Read the model definition and answer for the solid it produces. Units are mm, in the model's axes. Face numbers are marked on the shaded views. A direction names the side the tool comes from. Coordinates: 2 decimals unless noted, no trailing zeros. Loops run counter-clockwise (first coordinate to the right, second up) from the corner with the lowest first, then second, coordinate; pieces in that order, holes last. Notation, with made-up numbers: (63.25, 36) -> (71.25, 36) arc R18 ccw to (71.25, 41) -> close; hole circle Ø7 at (56.25, -1). An arc over 180 degrees is marked (long way). Answer as a JSON object with one key per item and string values. Group by question number.
Q1. The part is cut by section D-D on x = 9. Write down the section's boundary in (y, z), and give its area (3 significant figures).
Q2. Straight lines are drawn through the part: line 1 along X through (y, z) = (0.5, 1.25) (3 decimals); line 2 along Z through (x, y) = (7.25, 6.25); line 3 along X through (y, z) = (-2.5, -5.25) (3 decimals). For each, find the intervals that lie inside material, in ascending order. Write a range as [from, to].
Q3. Determine the mould class of the marked faces 1, 2 and 3 for opening direction X: released by +X, released by -X, zero draft, split by the parting line, or undercut.
Q4. For the marked faces 4, 5 and 6, determine the directions among +Z, -Z, +X, -X, +Y, -Y from which every point of the face is accessible in a straight line to the end or side of a thin tool.
Q5. The part is cut by section A-A on z = 1. Write down the section's boundary in (x, y) (3 decimals), and give its area (3 significant figures).
Q6. The part is cut by section C-C on y = 3. Write down the section's boundary in (x, z) (3 decimals), and give its area (3 significant figures).
Q7. Each of these flat-tipped pins is pushed along its axis until it touches: P1, Ø3, axis at x = 9, y = 4.5, coming from the +Z side; P2, Ø1.1, axis at x = -12, z = 1, coming from the +Y side (3 decimals); P3, Ø1.5, axis at x = 12, z = 1.5, coming from the -Y side (3 decimals). Where does it stop, or does it pass through?
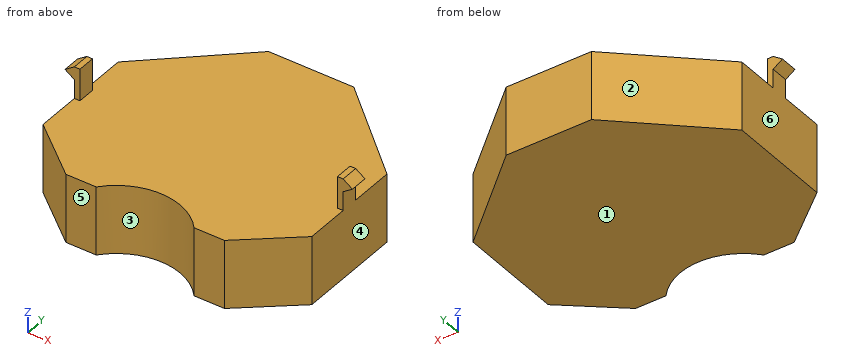
from build123d import *

# Parameters (mm, degrees)
F1_DEPTH      = 6.1
F3_DEPTH      = 0.785
F3_DEPTH_BACK = 0.785
F5_DEPTH      = 8.931
F6_ANGLE      = 180


with BuildPart() as f1:
    # F0 (on Top) → F1 (new body)
    with BuildSketch(Plane.XY):
        Polygon((-7.0355, 8.75), (-11.925, 4.7117), (-11.925, -4.7117), (-3.785, -12.05), (3.785, -12.05), (11.925, -4.7117), (11.925, 4.7117), (7.0355, 8.75), align=None)
    extrude(amount=F1_DEPTH)

    # F2 (on Front) → F3 (join, two sides)
    with BuildSketch(Plane.XZ) as f3_sk:
        Polygon((-11.425, 0), (-11.925, 0), (-11.925, -1.6852878034), (-12.75, -2.2576439017), (-11.925, -2.83), (-11.425, -2.83), align=None)
        Polygon((11.925, -1.6852878034), (11.925, 0), (11.425, 0), (11.425, -2.83), (11.925, -2.83), (12.75, -2.2576439017), align=None)
    extrude(amount=F3_DEPTH)
    extrude(f3_sk.sketch, amount=-F3_DEPTH_BACK)

    # F4 (on face) → F5 (cut, through all)
    with BuildSketch(Plane.XY.offset(6.1)):
        with BuildLine():
            Line((4.342041453, 8.75), (-4.342041453, 8.75))
            ThreePointArc((-4.342041453, 8.75), (0, 6.7139288477), (4.342041453, 8.75))
        make_face()
    extrude(amount=-F5_DEPTH, mode=Mode.SUBTRACT)


with BuildPart() as f1_1:
    # F6: moved
    add(f1.part.rotate(Axis((-2.2744432418, 0, 0), (1, 0, 0)), F6_ANGLE))


solid = f1_1.part
Final values:
{
 "1": {"outline": "(-7.13, -6.1) -> (7.35, -6.1) -> (7.35, 0) -> (-7.13, 0) -> close", "area": "88.3 mm2"},
 "2": {"line 1": "x = [-11.925, -11.425], [11.425, 11.925]", "line 2": "z = [-6.1, 0]", "line 3": "x = [-11.925, 11.925]"},
 "3": {"face 1": "zero draft", "face 2": "released by -X", "face 3": "undercut"},
 "4": {"face 4": "-Z, +X, +Y, -Y", "face 5": "+Z, -Z, +X, -X, -Y", "face 6": "-Z, -X, +Y, -Y"},
 "5": {"outline": "(-11.925, -0.785) -> (-11.425, -0.785) -> (-11.425, 0.785) -> (-11.925, 0.785) -> close; (11.425, -0.785) -> (11.925, -0.785) -> (11.925, 0.785) -> (11.425, 0.785) -> close", "area": "1.57 mm2"},
 "6": {"outline": "(-11.925, -6.1) -> (11.925, -6.1) -> (11.925, 0) -> (-11.925, 0) -> close", "area": "145 mm2"},
 "7": {"P1": "stops at z = 0", "P2": "stops at y = 0.785", "P3": "stops at y = -0.785"}
}
